Geometry check sheet. Reference: the model listing, model coordinates, mm. A direction names the side the tool comes from. Give positions to 0.01 mm unless a question says otherwise; leave off trailing zeros. Loops run counter-clockwise (first coordinate to the right, second up) from the corner with the lowest first, then second, coordinate; pieces in that order, holes last. Notation, with made-up numbers: (54.5, 65) -> (99.5, 65) arc R4 cw to (99.5, 69) -> close; hole circle Ø3 at (-27.5, 18.25). An arc over 180 degrees is marked (long way). Write item = value, one per line.
```python
from build123d import *

# Parameters (mm, degrees)
F1_DEPTH = 25
F2_D     = 5.1


# Not quite as in the source:
# - a feature names something its author has since deleted; it is built from what else it names


with BuildPart() as f1:
    # F0 (on Right) → F1 (new body)
    with BuildSketch(Plane.YZ):
        Polygon((24.1157077886, 30.274353966), (19.0699821276, 30.274353966), (19.0699821276, 0), (49.3443360936, 0), (49.3443360936, 30.274353966), (44.2986104326, 30.274353966), (34.2071591106, 20.182902644), align=None)
    extrude(amount=F1_DEPTH)

    # F2 (through all)
    with Locations(Plane(origin=(0, 0, 0), x_dir=(0, 1, 0), z_dir=(-1, 0, 0))):
        with Locations((34.2071591106, -5), (34.2071591106, -15.137176983)):
            Hole(F2_D / 2)


solid = f1.part
```
Item 1: Section check B-B, the plane x = 18.25. Record the cut outline in (y, z).
Answer:
outline = (19.07, 0) -> (49.34, 0) -> (49.34, 30.27) -> (44.3, 30.27) -> (34.21, 20.18) -> (24.12, 30.27) -> (19.07, 30.27) -> close; hole circle Ø5.1 at (34.21, 5); hole circle Ø5.1 at (34.21, 15.14)
Item 2: Gauge pin test, flat ends, axial feed: pin 1 (5 mm diameter, centred on x = 10.5, y = 29.5, fed in from +Z); pin 2 (4.5 mm diameter, centred on y = 34.21, z = 5, fed in from +X). Record the tip position at first contact, or that the pin passes through.
Answer:
pin_1 = 27.39
pin_2 = through
Item 3: Section check A-A, the plane z = 5. Record the cut outline in (x, y), plus the area to 3 significant figures.
Answer:
outline = (0, 19.07) -> (25, 19.07) -> (25, 31.66) -> (0, 31.66) -> close; (0, 36.76) -> (25, 36.76) -> (25, 49.34) -> (0, 49.34) -> close
area = 629 mm^2
Item 4: Draft check along Y on faces 3 (the flat face through (0, 34, 12)), 4 (the flat face through (12.32, 29.23, 25.16)), 5 (the flat face through (12, 49.344, 15)). Enter one of: +Y half, -Y half, draft (parallel to the pull), parting line (faces both ways), or undercut.
Answer:
face_3 = draft
face_4 = undercut
face_5 = +Y half
Item 5: Section check C-C, the plane z = 22.5. Record the cut outline in (x, y).
Answer:
outline = (0, 19.07) -> (25, 19.07) -> (25, 31.89) -> (0, 31.89) -> close; (0, 36.52) -> (25, 36.52) -> (25, 49.34) -> (0, 49.34) -> close
Item 6: Section check D-D, the plane y = 30. Record the cut outline in (x, z).
Answer:
outline = (0, 0) -> (25, 0) -> (25, 24.39) -> (0, 24.39) -> close
Item 7: Tool access check on faces 1 (the cylindrical face through (12.675, 36.755, 4.888)), 2 (the flat face through (12.325, 39.324, 25.299)). Record the directions out of +Z, -Z, +X, -X, +Y, -Y that give a thin tool (end or side, any length) a straight path to the whole face; none if there is none.
Answer:
face_1 = +X, -X
face_2 = +Z, +X, -X
Item 8: Thickness scan on L1, parallel to Z at x = 15.5, y = 35.5; L2, parallel to Z at x = 17.75, y = 36; L3, parallel to Y at x = 8.75, z = 4.5. Record the ranges inside material, lowest first. Write a range as [from, to].
Answer:
L1 = [0, 2.8], [7.2, 12.94], [17.34, 21.48]
L2 = [0, 3.19], [6.81, 13.32], [16.95, 21.98]
L3 = [19.07, 31.71], [36.71, 49.34]
